```python
from build123d import *

# Parameters (mm, degrees)
BOSS_EXTRUDE1_DEPTH     = 33
CHAMFER1_SIZE           = 1.5
G1_8_TAPPED_HOLE1_D     = 4.2
G1_8_TAPPED_HOLE1_DEPTH = 11
G1_8_TAPPED_HOLE1_TIP   = 1.2618073
SKETCH6_R               = 3
CUT_EXTRUDE1_DEPTH      = 34


with BuildPart() as part:
    # Sketch1 → Boss-Extrude1 (new body)
    with BuildSketch(Plane(origin=(0, 0, 0), x_dir=(0, 0, -1), z_dir=(1, 0, 0))):
        with BuildLine():
            Line((-4.85, 8.745141508), (-4.85, 10.5))
            Line((-4.85, 10.5), (4.85, 10.5))
            Line((4.85, 10.5), (4.85, 8.745141508))
            ThreePointArc((4.85, 8.745141508), (0, -10), (-4.85, 8.745141508))
        make_face()
    extrude(amount=BOSS_EXTRUDE1_DEPTH)

    # Sketch2 → Cut-Revolve1 (revolve, cut)
    with BuildSketch(Plane.XY):
        Polygon((27, 14), (27, 6.75), (28.35, 6.75), (28.35, 6), (33, 6), (33, 14), align=None)
    revolve(axis=Axis((45.5, 0, 0), (-1, 0, 0)), mode=Mode.SUBTRACT)

    # Sketch3 → Cut-Revolve2 (revolve, cut)
    with BuildSketch(Plane.XY):
        Polygon((0, 8), (15, 8), (15.5, 7.5), (17, 7.5), (17, 16), (0, 16), align=None)
    revolve(axis=Axis((0, 0, 0), (1, 0, 0)), mode=Mode.SUBTRACT)

    # Chamfer1
    chamfer1_edges = [part.edges().sort_by_distance(p)[0] for p in [
        (0, -8, 0),
    ]]
    chamfer(chamfer1_edges, length=CHAMFER1_SIZE)

    # G1/8 Tapped Hole1
    with Locations(Plane(origin=(0, 10.5, 0), x_dir=(-1, 0, 0), z_dir=(0, 1, 0))):
        with Locations((-23, 0)):
            Hole(G1_8_TAPPED_HOLE1_D / 2, depth=G1_8_TAPPED_HOLE1_DEPTH)
            with Locations((0, 0, -(G1_8_TAPPED_HOLE1_DEPTH + G1_8_TAPPED_HOLE1_TIP / 2))):  # 118° drill point
                Cone(0, G1_8_TAPPED_HOLE1_D / 2, G1_8_TAPPED_HOLE1_TIP, mode=Mode.SUBTRACT)

    # Sketch6 → Cut-Extrude1 (cut, through all)
    with BuildSketch(Plane(origin=(33, 0, 0), x_dir=(0, 0, -1), z_dir=(1, 0, 0))):
        Circle(SKETCH6_R)
    extrude(amount=-CUT_EXTRUDE1_DEPTH, mode=Mode.SUBTRACT)


solid = part.part
```
Geometry: final body of the model. Coordinates: model frame, mm. A direction names the side the tool comes from. Coordinates: 2 decimals unless noted, no trailing zeros. Write each loop counter-clockwise with the first axis right and the second up, starting at its lowest first coordinate (ties: lowest second). Pieces come first, ordered by that corner, then holes. Notation, with made-up numbers: M 39,30 L 60,30 A18 ccw 60,39 Z; hole C -39.5,85 d3. An arc over 180 degrees is marked long. Answer as CSV lines item,"result". Start each with the question number.
Q1. Mould query, pull axis Y, two halves, no side actions, for faces 1 (the cylindrical face through (16.73, -2.93, 0.65)), 2 (the flat face through (22, 10, -4.85)), 3 (the flat face through (20.8, 10.5, 1.1)). Classes: released by +Y, released by -Y, zero draft, split by the parting line, or undercut.
Q2. Reachability of faces 4 (the cylindrical face through (27.68, -1.46, 6.59)), 5 (the flat face through (22, 10, 4.85)), 6 (the flat face through (17, 5, -7)), 7 (the cylindrical face through (25.003, 6.263, 0.631)), 8 (the cylindrical face through (8.34, -1.73, -7.81)) from +Z, -Z, +X, -X, +Y, -Y: full face, straight path, thin tool, end or side. Return the list, or none.
Q3. Pin query (flat end, axial travel): P1, Ø1.9, axis at x = 23, y = 9.5, coming from the -Z side; P2, Ø1.9, axis at x = 24, y = 9.5, coming from the +Z side; P3, Ø8, axis at x = 16, y = -5.5, coming from the +Z side. Return the tip coordinate at first contact, or that it passes through.
Q4. Cut plane A-A on y = 0. Return the cut outline in (x, z).
Q5. Line query: line 1 (X direction, y = 7.75, z = 0); line 2 (X direction, y = 6.5, z = 6.75); line 3 (Z direction, x = 28, y = 2.5). Output: solid intervals per line, ascending. Write a range as from..to.
Q6. Cut plane B-B on z = 0. Count the separate pieces of the cut face and the enclosed holes in it, then the cut area to 3 significant figures.
Q7. Cut plane C-C on x = 26. Return the cut outline in (y, z).
Q8. Cut plane D-D on x = 16. Return the cut outline in (y, z).
Findings below:
1,face 1,"undercut"
1,face 2,"zero draft"
1,face 3,"released by +Y"
2,face 4,"+X"
2,face 5,"+Z, +X, -X, +Y"
2,face 6,"none"
2,face 7,"+Y"
2,face 8,"-X"
3,P1,"stops at z = -5.19"
3,P2,"stops at z = 5.19"
3,P3,"stops at z = 9.87"
4,outline,"M 0,-6.5 L 1.5,-8 L 15,-8 L 15.5,-7.5 L 17,-7.5 L 17,-10 L 27,-10 L 27,-6.75 L 28.35,-6.75 L 28.35,-6 L 33,-6 L 33,-3 L 0,-3 Z; M 0,3 L 33,3 L 33,6 L 28.35,6 L 28.35,6.75 L 27,6.75 L 27,10 L 17,10 L 17,7.5 L 15.5,7.5 L 15,8 L 1.5,8 L 0,6.5 Z"
5,line 1,"x = 1.25..15.25, 17..20.9, 25.1..27"
5,line 2,"x = 17..27"
5,line 3,"z = -6.27..-1.66, 1.66..6.27"
6,separate pieces,"3"
6,enclosed holes,"0"
6,area,"318 mm2"
7,outline,"M 8.75,-4.85 L 10.5,-4.85 L 10.5,4.85 L 8.75,4.85 A10 ccw long Z; hole C 0,0 d6"
8,outline,"C 0,0 d15; hole C 0,0 d6"
